from build123d import *

# Parameters (mm, degrees)
F1_DEPTH = 12.7
F2_SIZE  = 5.07999


# Not quite as in the source:
# - a fillet or chamfer is up to 0.001 mm smaller than in the source, because OpenCascade refuses the exact size


with BuildPart() as f1:
    # F0 (on Front) → F1 (new body)
    with BuildSketch(Plane.XZ):
        Polygon((-7.1858047352, 75.0022197947), (-7.1858047352, 7.1842197947), (-55.1002257696, -40.8236010231), (-47.909149441, -48.0009279096), (0, 0), (48.0004344931, -47.9086569679), (55.1777613797, -40.7175806394), (7.1841965553, 7.1842197947), (7.1841965553, 75.0022197947), align=None)
    extrude(amount=F1_DEPTH)

    # F2 (size 5.08 in the source; OpenCascade refuses exactly that, so slightly less here)
    f2_edges = [f1.edges().sort_by_distance(p)[0] for p in [
        (7.184197, -12.7, 41.09322),
        (-0.000804, -12.7, 75.00222),
        (-7.185805, -12.7, 41.09322),
        (-31.143015, -12.7, -16.819691),
        (-51.504688, -12.7, -44.412264),
        (-23.954575, -12.7, -24.000464),
        (24.000217, -12.7, -23.954328),
        (51.589098, -12.7, -44.313119),
        (31.180979, -12.7, -16.76668),
    ]]
    chamfer(f2_edges, length=F2_SIZE)


solid = f1.part
Input: part model. Units: mm. Frame: model coordinates. A direction names the side the tool comes from. Coordinates: 2 decimals unless noted, no trailing zeros. Order: outer loops, then holes, each group sorted by start corner. A loop starts at its lowest first (then second) coordinate and runs counter-clockwise, first axis right, second up.
1. Ray query, line 1 along X through (y, z) = (-3.25, 38); line 2 along X through (y, z) = (-11.5, 1.5); line 3 along X through (y, z) = (-8, -7). Return the intervals inside material, ascending.
Checked values:
line 1: x = -7.19 to 7.18
line 2: x = -7.38 to -3.98, 3.99 to 7.39
line 3: x = -20.81 to -7.52, 7.55 to 20.86
2. Draft query along X for faces 1 (the flat face through (0.1, -9.63, 72.99)), 2 (the flat face through (23.664, -3.757, -23.619)), 3 (the flat face through (28.962, -10.196, -18.191)). Return one class per face: +X half, -X half, draft (parallel to the pull), parting line (faces both ways), or undercut.
Checked values:
face 1: draft
face 2: undercut
face 3: +X half
3. Cut plane A-A, the plane y = -5.5. Return loops of the section in (x, z), plus the area to 3 significant figures.
Checked values:
outline: (-55.1, -40.82) - (-47.91, -48) - (0, 0) - (48, -47.91) - (55.18, -40.72) - (7.18, 7.18) - (7.18, 75) - (-7.19, 75) - (-7.19, 7.18) - close
area: 2,400 mm2
4. Cut plane D-D, the plane z = 35.5. Return loops of the section in (x, y).
Checked values:
outline: (-7.19, -7.62) - (-2.11, -12.7) - (2.1, -12.7) - (7.18, -7.62) - (7.18, 0) - (-7.19, 0) - close
5. Access query for faces 4 (the flat face through (7.184, -4, 41)), 5 (the flat face through (4.609, -10.196, 39.55)), 6 (the flat face through (-24.344, -10.196, -20.744)). Directions: +Z, -Z, +X, -X, +Y, -Y. A direction counts if a zero-diameter tool reaches every point of the face in a straight line with its end or side. Return the directions, or none.
Checked values:
face 4: +Z, +X, +Y, -Y
face 5: +Z, +X, -Y
face 6: -Z, -Y
6. Contact query for flat-ended pins moving along their axis: P1, Ø4, axis at x = 25.5, y = -3.5, coming from the -Z side; P2, Ø3, axis at x = 35.5, y = -2.5, coming from the +Z side; P3, Ø1.5, axis at y = -8.5, z = 34, coming from the -X side. Output: stop coordinate, or through.
Checked values:
P1: stops at z = -27.45
P2: stops at z = -19.58
P3: stops at x = -7.06
